```python
from build123d import *

# Parameters (mm, degrees)
CROQUIS1_W              = 22
CROQUIS1_H              = 6.35
SALIENTE_EXTRUIR1_DEPTH = 2.8067
CROQUIS2_W              = 2.5
CROQUIS2_H              = 0.224358974
SALIENTE_EXTRUIR2_DEPTH = 1.07696
SALIENTE_EXTRUIR2_TAPER = 3
REDONDEO1_R             = 0.049609375
CORTAR_EXTRUIR1_DEPTH   = 13.798873245


with BuildPart() as part:
    # Croquis1 → Saliente-Extruir1 (new body)
    with BuildSketch(Plane(origin=(0, 0, 0), x_dir=(1, 0, 0), z_dir=(0, 1, 0))):
        Rectangle(CROQUIS1_W, CROQUIS1_H)
    extrude(amount=SALIENTE_EXTRUIR1_DEPTH)

    # Croquis2 → Saliente-Extruir2 (add)
    with BuildSketch(Plane.ZY.offset(11)):
        with Locations((0, 1.397)):
            Rectangle(CROQUIS2_W, CROQUIS2_H)
    extrude(amount=SALIENTE_EXTRUIR2_DEPTH, taper=SALIENTE_EXTRUIR2_TAPER)

    # Chaflán1: read off the stored shape, not the designer's step
    # Chaflán1: loft between two sections, ruled curve by curve
    chafl_n1_from = [
        Edge.make_line((-12.07696, 1.34070485, -1.194115663), (-12.07696, 1.34070485, 1.194115663)),
        Edge.make_line((-12.07696, 1.34070485, 1.194115663), (-12.07696, 1.45329515, 1.194115663)),
        Edge.make_line((-12.07696, 1.34070485, -1.194115663), (-12.07696, 1.45329515, -1.194115663)),
        Edge.make_line((-12.07696, 1.45329515, 1.194115663), (-12.07696, 1.45329515, -1.194115663)),
    ]
    chafl_n1_to = [
        Edge.make_line((-11, 0.718921704, -1.815898809), (-11, 0.718921704, 1.815898809)),
        Edge.make_line((-11, 0.718921704, 1.815898809), (-11, 2.075078296, 1.815898809)),
        Edge.make_line((-11, 0.718921704, -1.815898809), (-11, 2.075078296, -1.815898809)),
        Edge.make_line((-11, 2.075078296, 1.815898809), (-11, 2.075078296, -1.815898809)),
    ]
    chafl_n1 = Solid(Shell([*[Face.make_surface_from_curves(chafl_n1_from[k], chafl_n1_to[k]) for k in range(4)], Face(Wire(chafl_n1_from)), Face(Wire(chafl_n1_to))]))
    add(chafl_n1)

    # Redondeo1
    redondeo1_edges = [part.edges().sort_by_distance(p)[0] for p in [
        (-11.53848, 1.029813277, 1.505007236),
        (-11.53848, 1.029813277, -1.505007236),
        (-11.53848, 1.764186723, 1.505007236),
        (-11.53848, 1.764186723, -1.505007236),
    ]]
    fillet(redondeo1_edges, radius=REDONDEO1_R)

    # Croquis4 → Cortar-Extruir1 (cut, through all)
    with BuildSketch(Plane.XZ):
        with BuildLine():
            Line((-12.07696, -1.194115663), (-12.07696, 1.194115663))
            ThreePointArc((-12.07696, 1.194115663), (-11.963672899, 0), (-12.07696, -1.194115663))
        make_face()
    extrude(amount=-CORTAR_EXTRUIR1_DEPTH, mode=Mode.SUBTRACT)


solid = part.part
```
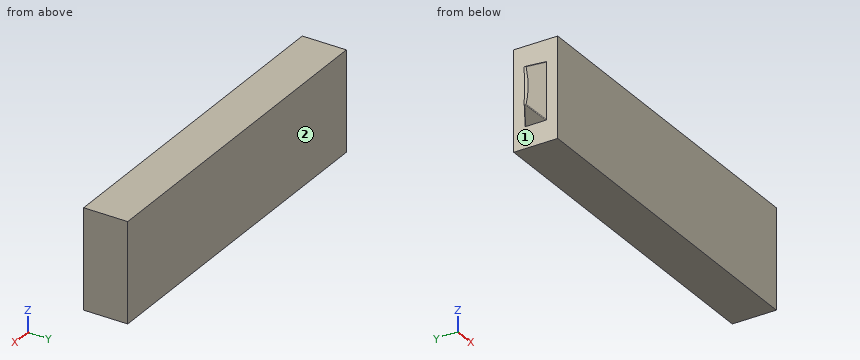
Source: CAD feature listing. Evaluate the final solid. Frame: model axes, mm. Face numbers are marked on the shaded views. A direction names the side the tool comes from. Round coordinates to 2 decimals unless told otherwise and drop trailing zeros. Loops run counter-clockwise (first coordinate to the right, second up) from the corner with the lowest first, then second, coordinate; pieces in that order, holes last. Notation, with made-up numbers: M 83,75.25 L 102,75.25 A11 ccw 102,80.25 Z; hole C 7,-23 d11. An arc over 180 degrees is marked long. Use a Markdown table: item, result. Add a question column.
1. Set-up query: the marked faces 1 and 2. Return all of +Z, -Z, +X, -X, +Y, -Y with unobstructed straight access to the full face (end or side cutting, diameter ignored); none if empty.
2. Cut plane B-B, the plane z = 2.5. Output: boundary loops of the cut face in (x, y), and give its area (3 significant figures).
3. Ray query, line 1 along X through (y, z) = (0.55, 1.25); line 2 along X through (y, z) = (1.2, 0). Return the intervals inside material, ascending. Write a range as [from, to].
4. Cut plane A-A, the plane y = 0.3. Output: boundary loops of the cut face in (x, z) (3 decimals), and give its area (3 significant figures).
Solution:
| question | item | result |
|---|---|---|
| 1 | face 1 | -X |
| 1 | face 2 | +Z, -Z, +X, -X, +Y |
| 2 | outline | M -11,0 L 11,0 L 11,2.81 L -11,2.81 Z |
| 2 | area | 61.7 mm2 |
| 3 | line 1 | x = [-11, 11] |
| 3 | line 2 | x = [-11.83, 11] |
| 4 | outline | M -11,-3.175 L 11,-3.175 L 11,3.175 L -11,3.175 Z |
| 4 | area | 140 mm2 |
